Could you check a few things on this model? Use its own coordinates, in mm. Give positions to 0.01 mm unless a question says otherwise; leave off trailing zeros. Answer in a Markdown table with one row per item. Add a question column.
```python
from build123d import *

# Parameters (mm, degrees)
SKETCH_W  = 10
SKETCH_H  = 6
PAD_DEPTH = 1


with BuildPart() as part:
    # Sketch → Pad (new body)
    with BuildSketch(Plane.XY):
        Polygon((-5, 5.886205), (5, 5.886205), (5, 0.113795), (6, 0.113795), (6, 244.227589), (5, 244.227589), (5, 238), (-5, 238), (-5, 244), (-6, 244), (-6, -0.113795), (-5, -0.113795), align=None)
        with Locations((0, 16.886205)):
            Rectangle(SKETCH_W, SKETCH_H, mode=Mode.SUBTRACT)
        with Locations((0, 24)):
            Rectangle(SKETCH_W, SKETCH_H, mode=Mode.SUBTRACT)
        with Locations((0, 31)):
            Rectangle(SKETCH_W, SKETCH_H, mode=Mode.SUBTRACT)
        with Locations((0, 38)):
            Rectangle(SKETCH_W, SKETCH_H, mode=Mode.SUBTRACT)
        with Locations((0, 45)):
            Rectangle(SKETCH_W, SKETCH_H, mode=Mode.SUBTRACT)
        with Locations((0, 52)):
            Rectangle(SKETCH_W, SKETCH_H, mode=Mode.SUBTRACT)
        with Locations((0, 59)):
            Rectangle(SKETCH_W, SKETCH_H, mode=Mode.SUBTRACT)
        with Locations((0, 66)):
            Rectangle(SKETCH_W, SKETCH_H, mode=Mode.SUBTRACT)
        with Locations((0, 73)):
            Rectangle(SKETCH_W, SKETCH_H, mode=Mode.SUBTRACT)
        with Locations((0, 80)):
            Rectangle(SKETCH_W, SKETCH_H, mode=Mode.SUBTRACT)
        with Locations((0, 87)):
            Rectangle(SKETCH_W, SKETCH_H, mode=Mode.SUBTRACT)
        with Locations((0, 94)):
            Rectangle(SKETCH_W, SKETCH_H, mode=Mode.SUBTRACT)
        with Locations((0, 101)):
            Rectangle(SKETCH_W, SKETCH_H, mode=Mode.SUBTRACT)
        with Locations((0, 108)):
            Rectangle(SKETCH_W, SKETCH_H, mode=Mode.SUBTRACT)
        with Locations((0, 115)):
            Rectangle(SKETCH_W, SKETCH_H, mode=Mode.SUBTRACT)
        with Locations((0, 122)):
            Rectangle(SKETCH_W, SKETCH_H, mode=Mode.SUBTRACT)
        with Locations((0, 129)):
            Rectangle(SKETCH_W, SKETCH_H, mode=Mode.SUBTRACT)
        with Locations((0, 136)):
            Rectangle(SKETCH_W, SKETCH_H, mode=Mode.SUBTRACT)
        with Locations((0, 143)):
            Rectangle(SKETCH_W, SKETCH_H, mode=Mode.SUBTRACT)
        with Locations((0, 150)):
            Rectangle(SKETCH_W, SKETCH_H, mode=Mode.SUBTRACT)
        with Locations((0, 157)):
            Rectangle(SKETCH_W, SKETCH_H, mode=Mode.SUBTRACT)
        with Locations((0, 164)):
            Rectangle(SKETCH_W, SKETCH_H, mode=Mode.SUBTRACT)
        with Locations((0, 171)):
            Rectangle(SKETCH_W, SKETCH_H, mode=Mode.SUBTRACT)
        with Locations((0, 178)):
            Rectangle(SKETCH_W, SKETCH_H, mode=Mode.SUBTRACT)
        with Locations((0, 185)):
            Rectangle(SKETCH_W, SKETCH_H, mode=Mode.SUBTRACT)
        with Locations((0, 192)):
            Rectangle(SKETCH_W, SKETCH_H, mode=Mode.SUBTRACT)
        with Locations((0, 199)):
            Rectangle(SKETCH_W, SKETCH_H, mode=Mode.SUBTRACT)
        with Locations((0, 206)):
            Rectangle(SKETCH_W, SKETCH_H, mode=Mode.SUBTRACT)
        with Locations((0, 213)):
            Rectangle(SKETCH_W, SKETCH_H, mode=Mode.SUBTRACT)
        with Locations((0, 220)):
            Rectangle(SKETCH_W, SKETCH_H, mode=Mode.SUBTRACT)
        with Locations((0, 227)):
            Rectangle(SKETCH_W, SKETCH_H, mode=Mode.SUBTRACT)
        with Locations((0, 234)):
            Rectangle(SKETCH_W, SKETCH_H, mode=Mode.SUBTRACT)
        with Locations((0, 9.886205)):
            Rectangle(SKETCH_W, SKETCH_H, mode=Mode.SUBTRACT)
    extrude(amount=PAD_DEPTH)


solid = part.part
```
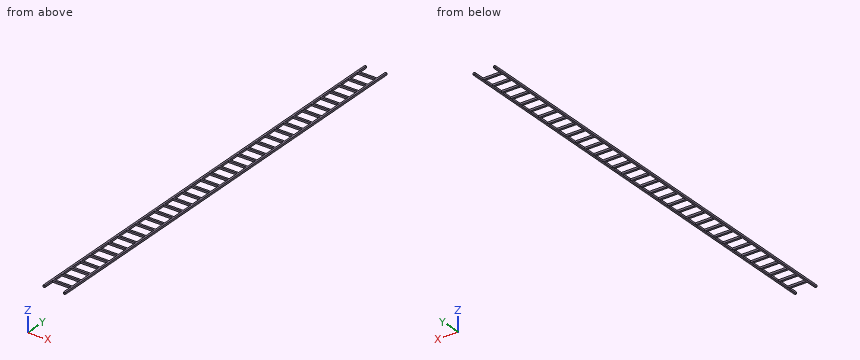
1. Suppose I cut it at A-A on z = 0.65. Count the separate pieces of the cut face and the enclosed holes in it, plus the area to 3 significant figures.
2. If I drill on line 1 along X through (y, z) = (127, 0.7), over which ranges is the centre line in solid material (lowest first)? Write a range as [from, to].
3. Will these pins go through, and if not, where does the flat tip stop? P1, Ø2, axis at x = 3.5, y = 129, coming from the -Z side; P2, Ø0.5, axis at x = 5.5, z = 0.5, coming from the -Y side.
Findings below:
| question | item | result |
|---|---|---|
| 1 | separate pieces | 1 |
| 1 | enclosed holes | 33 |
| 1 | area | 829 mm2 |
| 2 | line 1 | [-6, -5], [5, 6] |
| 3 | P1 | through |
| 3 | P2 | y = 0.11 |
